Source: CAD feature listing. Evaluate the final solid. Frame: model axes, mm. A direction names the side the tool comes from. Give positions to 0.01 mm unless a question says otherwise; leave off trailing zeros. Order: outer loops, then holes, each group sorted by start corner. A loop starts at its lowest first (then second) coordinate and runs counter-clockwise, first axis right, second up. Notation, with made-up numbers: M 14.25,-30.5 L 32.25,-30.5 A20 ccw 32.25,4.5 Z; hole C 20,-15.75 d7. An arc over 180 degrees is marked long. Answer in a Markdown table with one row per item. Add a question column.
(1) Material intervals for line 1 along X through (y, z) = (42.5, 7.5); line 2 along Y through (x, z) = (0, 17.75); line 3 along X through (y, z) = (-2, 3.75), sorted ascending.
(2) Section query A-A, the plane y = -15. Return loops of the section in (x, z).
(3) Section query B-B, the plane x = -2.5. Return loops of the section in (y, z), plus the area to 3 significant figures.
(4) Set-up query: faces 4 (the face through (60, -25, 10)), 5 (the face through (40.666, -0.091, 11.928)), 6 (the face through (-13.77, -61.99, 22.78)). Return all of +Z, -Z, +X, -X, +Y, -Y with unobstructed straight access to the full face (end or side cutting, diameter ignored); none if empty.
(5) Section query C-C, the plane x = 27.5. Count the separate pieces of the cut face and the enclosed holes in it, plus the area to 3 significant figures.
(6) Pin query (flat end, axial travel): P1, Ø5, axis at x = 40.5, y = -49, coming from the +Z side; P2, Ø5, axis at x = -28.5, z = 18.5, coming from the -Y side; P3, Ø12, axis at y = -12.5, z = 6, coming from the +X side; P4, Ø6, axis at x = 13.5, z = 12, coming from the -Y side. Return the tip coordinate at first contact, or that it passes through.
(7) Mould query, pull axis Z, two halves, no side actions, for faces 1 (the face through (28.69, -28.82, 11.93)), 2 (the face through (14.1, -62.3, 20.5)), 3 (the face through (14, -14, 0)). Classes: pulls with the +Z half, pulls with the -Z half, needs draft (parallel to the pull), parting line crosses it, or undercut.
from build123d import *

# Parameters (mm, degrees)
F0_R            = 65
F0_R_2          = 17.5
F1_DEPTH        = 25
F9_DEPTH        = 25
F9_COPIES_COUNT = 8
F10_R           = 65
F10_R_2         = 63.5
F11_DEPTH       = 4.5


# Not quite as in the source:
# - a pattern or mirror of a feature is missing from the dataset's text; its kind, count and spacing are read off the source's solid


with BuildPart() as f1:
    # F0 (on Top) → F1 (new body)
    with BuildSketch(Plane.XY):
        Circle(F0_R)
        Circle(F0_R_2, mode=Mode.SUBTRACT)
    extrude(amount=F1_DEPTH)

    # F8 (on 3pt) → F9 (cut)
    with BuildSketch(Plane(origin=(0, 66.1453359033, 3.4796235199), x_dir=(-1, 0, 0), z_dir=(0, 0.998619184, 0.0525330887))):
        with BuildLine():
            ThreePointArc((0, 3.1838245746), (4.5961940777, 5.0876304969), (6.5, 9.6838245746))
            ThreePointArc((6.5, 9.6838245746), (-4.5961940777, 14.2800186523), (0, 3.1838245746))
        make_face()
    f9 = extrude(amount=-F9_DEPTH, mode=Mode.SUBTRACT)

    # F9_copies: F9 ×8 about axis
    f9_copies_axis = Axis((0, 0, 0), (0, 0, 1))
    for i in range(1, F9_COPIES_COUNT):
        add(f9.rotate(f9_copies_axis, i * 360 / F9_COPIES_COUNT), mode=Mode.SUBTRACT)

    # F10 (on face) → F11 (cut)
    with BuildSketch(Plane.XY.offset(25)):
        Circle(F10_R)
        Circle(F10_R_2, mode=Mode.SUBTRACT)
    extrude(amount=-F11_DEPTH, mode=Mode.SUBTRACT)


solid = f1.part
Values follow:
| question | item | result |
|---|---|---|
| 1 | line 1 | x = -49.18 to -47.33, -36.88 to -4.76, 4.76 to 36.88, 47.33 to 49.18 |
| 1 | line 2 | y = -40.36 to -17.5, 17.5 to 40.36 |
| 1 | line 3 | x = -64.97 to -17.39, 17.39 to 64.97 |
| 2 | outline | M -63.25,0 L -9.01,0 L -9.01,25 L -61.7,25 L -61.7,20.5 L -63.25,20.5 Z; M 9.01,0 L 63.25,0 L 63.25,20.5 L 61.7,20.5 L 61.7,25 L 9.01,25 Z |
| 3 | outline | M -64.95,0 L -17.32,0 L -17.32,25 L -63.45,25 L -63.45,20.5 L -64.95,20.5 L -64.95,19.12 L -40.36,17.83 L -40.99,5.85 L -64.95,7.11 Z; M 17.32,0 L 64.95,0 L 64.95,7.11 L 40.99,5.85 L 40.36,17.83 L 64.95,19.12 L 64.95,20.5 L 63.45,20.5 L 63.45,25 L 17.32,25 Z |
| 3 | area | 1,780 mm² |
| 4 | face 4 | +Z, -Z |
| 4 | face 5 | none |
| 4 | face 6 | +Z |
| 5 | separate pieces | 1 |
| 5 | enclosed holes | 2 |
| 5 | area | 2,810 mm² |
| 6 | P1 | stops at z = 25 |
| 6 | P2 | stops at y = -59.57 |
| 6 | P3 | stops at x = 64.67 |
| 6 | P4 | stops at y = -64.15 |
| 7 | face 1 | undercut |
| 7 | face 2 | pulls with the +Z half |
| 7 | face 3 | pulls with the -Z half |
